Model file for the job. Use its own axes, mm. A direction names the side the tool comes from. Coordinates: 2 decimals unless noted, no trailing zeros. Loops run counter-clockwise (first coordinate to the right, second up) from the corner with the lowest first, then second, coordinate; pieces in that order, holes last. Notation, with made-up numbers: (54.5, 85.25) - (63.5, 85.25) arc R29 ccw to (63.5, 124.25) - close; hole circle Ø2 at (25, 81.5). An arc over 180 degrees is marked (long way). Write each question's results on one line, items separated by ' | '. Start each with the question number.
```python
from build123d import *

# Parameters (mm, degrees)
SKETCH_1_R          = 17
EXTRUDE_1_DEPTH     = 15
SKETCH_2_W          = 6
SKETCH_2_H          = 2
EXTRUDE_2_DEPTH     = 150
SKETCH_5_R          = 21
EXTRUDE_3_DEPTH     = 1.5
CUT_EXTRUDE_START   = -5
CUT_EXTRUDE_1_DEPTH = 5


with BuildPart() as part:
    # 草图1 → 凸台-拉伸1 (new body)
    with BuildSketch(Plane(origin=(0, 0, 0), x_dir=(1, 0, 0), z_dir=(0, 1, 0))):
        with Locations(Location((0, 0, 0), (0, 0, 270))):
            Circle(SKETCH_1_R)
    extrude(amount=EXTRUDE_1_DEPTH)

    # 草图2 → 切除-旋转1 (revolve, cut)
    with BuildSketch(Plane.XY, mode=Mode.PRIVATE) as cut_revolve_1_sk:
        with Locations((-14, 12)):
            Rectangle(SKETCH_2_W, SKETCH_2_H)
        with Locations((-14, 8)):
            Rectangle(SKETCH_2_W, SKETCH_2_H)
        with Locations((-14, 4)):
            Rectangle(SKETCH_2_W, SKETCH_2_H)
    revolve(cut_revolve_1_sk.sketch.rotate(Axis((0, 0, 0), (0, 1, 0)), 270), axis=Axis((0, 0, 0), (0, 1, 0)), mode=Mode.SUBTRACT)

    # 草图3 → 旋转2 (revolve)
    with BuildSketch(Plane.XY, mode=Mode.PRIVATE) as revolve_2_sk:
        Polygon((0, 0), (-17, 0), (0, -5), align=None)
    revolve(revolve_2_sk.sketch.rotate(Axis((0, 0, 0), (0, 1, 0)), 270), axis=Axis((0, 0, 0), (0, 1, 0)))

    # 草图4 → 凸台-拉伸2 (add)
    with BuildSketch(Plane(origin=(0, 15, 0), x_dir=(1, 0, 0), z_dir=(0, 1, 0))):
        with BuildLine():
            Line((-0.5, 16.992645468), (-0.5, 0.5))
            Line((-0.5, 0.5), (-16.992645468, 0.5))
            ThreePointArc((-16.992645468, 0.5), (-17, 0), (-16.992645468, -0.5))
            Line((-16.992645468, -0.5), (-0.5, -0.5))
            Line((-0.5, -0.5), (-0.5, -16.992645468))
            ThreePointArc((-0.5, -16.992645468), (0, -17), (0.5, -16.992645468))
            Line((0.5, -16.992645468), (0.5, -0.5))
            Line((0.5, -0.5), (16.992645468, -0.5))
            ThreePointArc((16.992645468, -0.5), (17, 0), (16.992645468, 0.5))
            Line((16.992645468, 0.5), (0.5, 0.5))
            Line((0.5, 0.5), (0.5, 16.992645468))
            ThreePointArc((0.5, 16.992645468), (0, 17), (-0.5, 16.992645468))
        make_face()
    extrude(amount=EXTRUDE_2_DEPTH)

    # 草图5 → 凸台-拉伸3 (add)
    with BuildSketch(Plane(origin=(0, 165, 0), x_dir=(1, 0, 0), z_dir=(0, 1, 0))):
        with Locations(Location((0, 0, 0), (0, 0, 270))):
            Circle(SKETCH_5_R)
    extrude(amount=EXTRUDE_3_DEPTH)

    # 草图7 → 切除-拉伸1 (cut)
    with BuildSketch(Plane(origin=(0, 166.5, 0), x_dir=(1, 0, 0), z_dir=(0, 1, 0)).offset(CUT_EXTRUDE_START)):
        with BuildLine():
            ThreePointArc((21, 0), (20.978166703, 0.957351445), (20.912712211, 1.912712211))
            Line((20.912712211, 1.912712211), (19, 0))
            Line((19, 0), (-1.912712211, -20.912712211))
            ThreePointArc((-1.912712211, -20.912712211), (14.156854234, -15.510753631), (21, 0))
        make_face()
        with BuildLine():
            Line((11.313708499, 13.435028843), (4.915542193, 7.036862537))
            ThreePointArc((4.915542193, 7.036862537), (4.915542193, 4.915542193), (7.036862537, 4.915542193))
            Line((7.036862537, 4.915542193), (13.435028843, 11.313708499))
            ThreePointArc((13.435028843, 11.313708499), (13.435028843, 13.435028843), (11.313708499, 13.435028843))
        make_face()
        with BuildLine():
            Line((1.912712211, 20.912712211), (-20.912712211, -1.912712211))
            ThreePointArc((-20.912712211, -1.912712211), (-14.849242405, 14.849242405), (1.912712211, 20.912712211))
        make_face()
    extrude(amount=CUT_EXTRUDE_1_DEPTH, mode=Mode.SUBTRACT)


solid = part.part
```
Q1. Pin check, flat tips, straight feed: pin 1 (5 mm diameter, centred on x = 14, y = 102.5, fed in from -Z); pin 2 (1.5 mm diameter, centred on y = 23.5, z = 12.5, fed in from -X); pin 3 (18 mm diameter, centred on y = 73, z = 5, fed in from -X). Stop position of each tip, or through.
Q2. Cut at B-B (x = -15). State how many separate pieces and enclosed holes the cut face has, and give its area (3 significant figures).
Q3. Cut at A-A (y = 20.5). List the corners of the cut face in (x, z).
Q4. Mould opens along Y. For faces 5 (the flat face through (-9, 166, -10)), 6 (the flat face through (11, 3, -4)), 7 (the flat face through (0.5, 89, 9)), 8 (the flat face through (0, 166.5, 0)) say: +Y half, -Y half, draft (parallel to the pull), parting line (faces both ways), or undercut.
Q5. Drill centre lines: L1, parallel to Y at x = 16, z = -5.5; L2, parallel to Y at x = 4.5, z = 15; L3, parallel to Y at x = -6.5, z = 13. Where is each one in solid material? Low to high. Write a range as from..to.
Q6. Which spindle directions (+Z, -Z, +X, -X, +Y, -Y) get a long thin tool onto all of the face, cutting with end or side? Do faces 1 (the flat face through (9, 89, 0.5)), 2 (the cylindrical face through (10.74, 8.01, 2.38)), 3 (the flat face through (7, 15, -7)), 4 (the cylindrical face through (16.855, 5.986, -2.213)). Say none if no direction does.
Check result:
1) pin 1: z = -0.5 | pin 2: x = -0.5 | pin 3: x = -17
2) separate pieces: 4 | enclosed holes: 0 | area: 328 mm²
3) outline: (-16.99, -0.5) - (-0.5, -0.5) - (-0.5, -16.99) arc R17 ccw to (0.5, -16.99) - (0.5, -0.5) - (16.99, -0.5) arc R17 ccw to (16.99, 0.5) - (0.5, 0.5) - (0.5, 16.99) arc R17 ccw to (-0.5, 16.99) - (-0.5, 0.5) - (-16.99, 0.5) arc R17 ccw to start
4) face 5: draft | face 6: undercut | face 7: undercut | face 8: +Y half
5) L1: -0.02..3, 5..7, 9..11, 13..15, 165..166.5 | L2: -0.39..3, 5..7, 9..11, 13..15 | L3: -0.73..3, 5..7, 9..11, 13..15, 165..166.5
6) face 1: +Z, +X | face 2: none | face 3: -Z, +X | face 4: -Y
